Part print with two shaded views. Sizes in mm from the minimum x, y, z corner. A direction names the side the tool comes from. Round coordinates to 2 decimals unless told otherwise and drop trailing zeros. Order: outer loops, then holes, each group sorted by start corner. A loop starts at its lowest first (then second) coordinate and runs counter-clockwise, first axis right, second up. Notation, with made-up numbers: M 17.5,53 L 24.5,53 A17 cw 24.5,71 Z; hole C 88,54 d3. An arc over 180 degrees is marked long. Put each result on its own line as item: value.
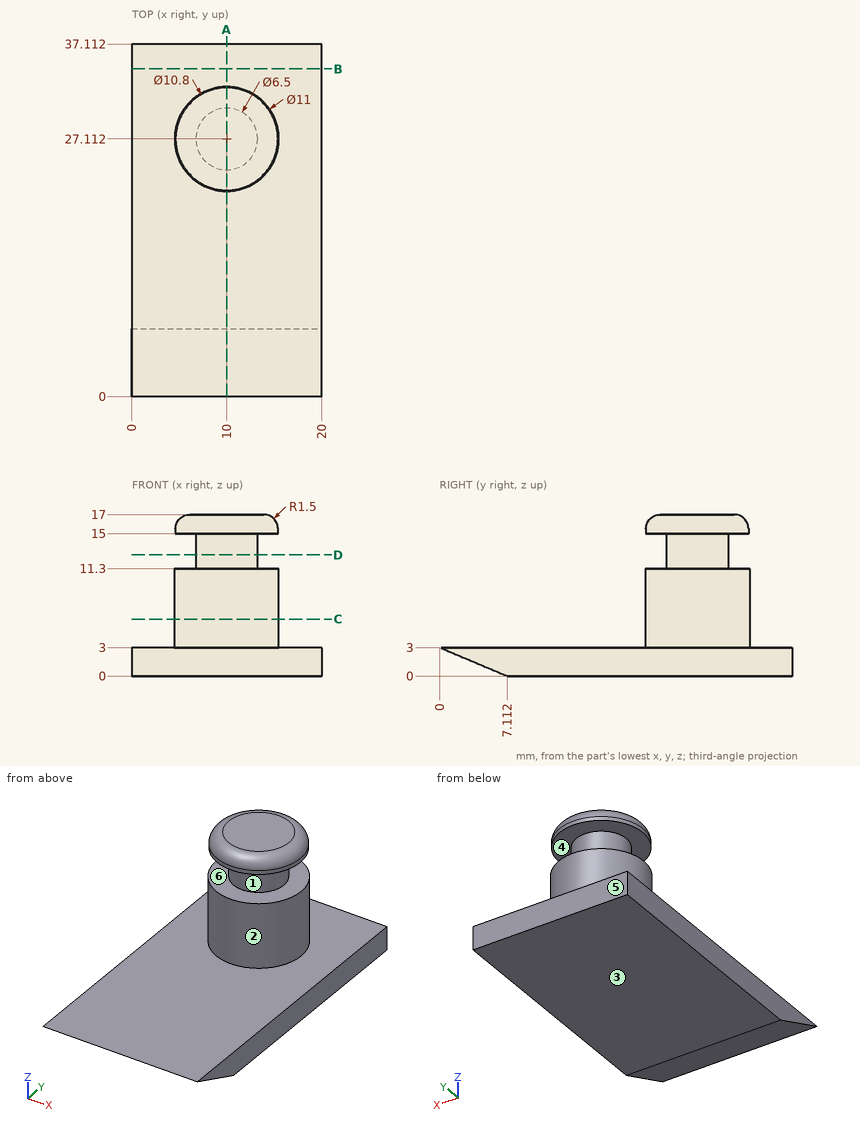
Item 1: Probe line 1 along Z through (x, y) = (10.25, 30.5); line 2 along Z through (x, y) = (5.25, 16.5); line 3 along X through (y, z) = (27, 3.5). List the from-to ranges inside material, lowest first. Write a range as [from, to].
Answers below:
line 1: [0, 11.3], [15, 17]
line 2: [0, 3]
line 3: [4.5, 15.5]
Item 2: Mould opens along Z. For the marked faces 1, 2, 3 and 4 say: pulls with the +Z half, pulls with the -Z half, needs draft (parallel to the pull), parting line crosses it, or undercut.
Answers below:
face 1: undercut
face 2: needs draft
face 3: pulls with the -Z half
face 4: undercut
Item 3: Band-saw the part on B-B on y = 34.5. Give the cut face in (x, z), and give its area (3 significant figures).
Answers below:
outline: M 0,0 L 20,0 L 20,3 L 0,3 Z
area: 60.0 mm²
Item 4: Band-saw the part on A-A on x = 10. Give the cut face in (y, z), and give its area (3 significant figures).
Answers below:
outline: M 0,3 L 7.11,0 L 37.11,0 L 37.11,3 L 32.61,3 L 32.61,11.3 L 30.36,11.3 L 30.36,15 L 32.51,15 L 32.51,15.5 A1.5 ccw 31.01,17 L 23.21,17 A1.5 ccw 21.71,15.5 L 21.71,15 L 23.86,15 L 23.86,11.3 L 21.61,11.3 L 21.61,3 Z
area: 237 mm²
Item 5: Tool access for the marked faces 5 and 6: list every direction of +Z, -Z, +X, -X, +Y, -Y with a clear straight run to the whole face (end or side of a thin tool).
Answers below:
face 5: +Z, -Z, +X, -X, +Y
face 6: none
Item 6: Band-saw the part on C-C on z = 6. Give the cut face in (x, y).
Answers below:
outline: C 10,27.11 d11
Item 7: Band-saw the part on D-D on z = 12.75. Give the cut face in (x, y).
Answers below:
outline: C 10,27.11 d6.5
Item 8: Pin check, flat tips, straight feed: P1, Ø1.5, axis at x = 2, y = 27, coming from the +Z side; P2, Ø5.5, axis at x = 9, y = 28.5, coming from the -Z side; P3, Ø10, axis at x = 17, z = 9.5, coming from the -Y side. Stop position of each tip, or through.
Answers below:
P1: z = 3
P2: z = 0
P3: y = 21.99
